```python
from build123d import *


with BuildPart() as f1:
    # F0 (on Front) → F1 (revolve)
    with BuildSketch(Plane.XZ):
        with BuildLine():
            Line((1.320192, 9.415357), (1.320192, 8.666018))
            Line((1.320192, 8.666018), (1.840662, 8.666018))
            Line((1.840662, 8.666018), (2.340662, 6.666018))
            Line((2.340662, 6.666018), (2.340662, 1.363074))
            Line((2.340662, 1.363074), (3.340662, 0.362162))
            Line((3.340662, 0.362162), (3.340662, -1.151177))
            Line((3.340662, -1.151177), (5.340662, -1.151177))
            Line((5.340662, -1.151177), (5.340662, 9.415357))
            Line((5.340662, 9.415357), (5.340662, 10.261006))
            Line((5.340662, 10.261006), (5.340662, 13.182231))
            Line((5.340662, 13.182231), (5.340662, 15.010567))
            ThreePointArc((5.340662, 15.010567), (2.779756, 13.190362), (3.656931, 10.173419))
            Line((3.656931, 10.173419), (3.656931, 9.415357))
            Line((3.656931, 9.415357), (1.320192, 9.415357))
        make_face()
    revolve(axis=Axis((5.340662, 0, 4.13209), (0, 0, 1)))


solid = f1.part
```
Design review of the part built by this model. Coordinates are the model's own, in mm. A direction names the side the tool comes from. Coordinates: 2 decimals unless noted, no trailing zeros. Loops run counter-clockwise (first coordinate to the right, second up) from the corner with the lowest first, then second, coordinate; pieces in that order, holes last.
Q1. For pin 1 (1.5 mm diameter, centred on y = 2.5, z = 2.5, fed in from +X); pin 2 (1.5 mm diameter, centred on y = -1, z = 10.5, fed in from +X); pin 3 (2 mm diameter, centred on x = 8, z = 3, fed in from +Y); pin 4 (2.5 mm diameter, centred on x = 6, y = -0.5, fed in from +Z), all flat-tipped, find the tip position at first contact; note any pin that passes through.
Reported:
pin 1: stops at x = 7.78
pin 2: stops at x = 7.72
pin 3: stops at y = 2.5
pin 4: stops at z = 15.01
Q2. We need section A-A on z = 5.5. State the section outline as (x, y) points, and give its area (3 significant figures).
Reported:
outline: circle Ø6 at (5.34, 0)
area: 28.3 mm2
Q3. Tool access review of faces 1 (the face through (5.864, -3.986, 9.035)), 2 (the face through (3.785, 0.645, 9.789)), 3 (the face through (5.774, 1.952, -0.405)): name each direction out of +Z, -Z, +X, -X, +Y, -Y from which nothing blocks a thin tool from reaching the whole face with its end or side.
Reported:
face 1: +Z, -Z
face 2: none
face 3: -Z
Q4. We need section B-B on z = 0. State the section outline as (x, y) points, and give its area (3 significant figures).
Reported:
outline: circle Ø4 at (5.34, 0)
area: 12.6 mm2
Q5. The part is to be moulded in two halves that separate along Z. For faces 4 (the face through (5, 2, 9.415)), 5 (the face through (2.48, -0.9, 3.98)), 6 (the face through (3, -3, 8.666)), say which applies: +Z half, -Z half, draft (parallel to the pull), parting line (faces both ways), or undercut.
Reported:
face 4: undercut
face 5: draft
face 6: -Z half
Q6. To check wall thickness, follow line 1 (Z direction, x = 3.5, y = -0.25); line 2 (Z direction, x = 5.25, y = 3.75); line 3 (Y direction, x = 5.5, z = 5.75). State the ranges of each line that lie inside material, in increasing order.
Reported:
line 1: z = -1.15 to 9.42, 10.32 to 14.27
line 2: z = 8.67 to 9.42
line 3: y = -3 to 3
